```python
from build123d import *

# Parameters (mm, degrees)
BLANKSKE_W         = 44.45
BLANKSKE_H         = 10.795
BLANK_DEPTH        = 9.525
TOOTHCUTSIM_DEPTH  = 47.723229233
TEETHCUTS_COUNT    = 12
TEETHCUTS_PITCH    = 3.989822666
SKETCH1_R          = 2.4892
CUT_EXTRUDE1_DEPTH = 14.478


with BuildPart() as part:
    # BlankSke → Blank (new body)
    with BuildSketch(Plane.XY):
        with Locations((22.225, 5.3975)):
            Rectangle(BLANKSKE_W, BLANKSKE_H)
    extrude(amount=-BLANK_DEPTH)

    # TooCutSkeSim → ToothCutSim (cut, through all)
    with BuildSketch(Plane.XY):
        Polygon((0.595165029, 8.001), (-0.595165029, 8.001), (-1.621342708, 10.8204), (1.621342708, 10.8204), align=None)
    toothcutsim = extrude(amount=-TOOTHCUTSIM_DEPTH, mode=Mode.SUBTRACT)

    # TeethCuts: ToothCutSim ×12
    with Locations(*[(i * TEETHCUTS_PITCH, 0, 0) for i in range(1, TEETHCUTS_COUNT)]):
        add(toothcutsim, mode=Mode.SUBTRACT)

    # Sketch1 → Cut-Extrude1 (cut)
    with BuildSketch(Plane.XY):
        with Locations((5.08, 4.0005)):
            Circle(SKETCH1_R)
    extrude(amount=-CUT_EXTRUDE1_DEPTH, mode=Mode.SUBTRACT)


solid = part.part
```
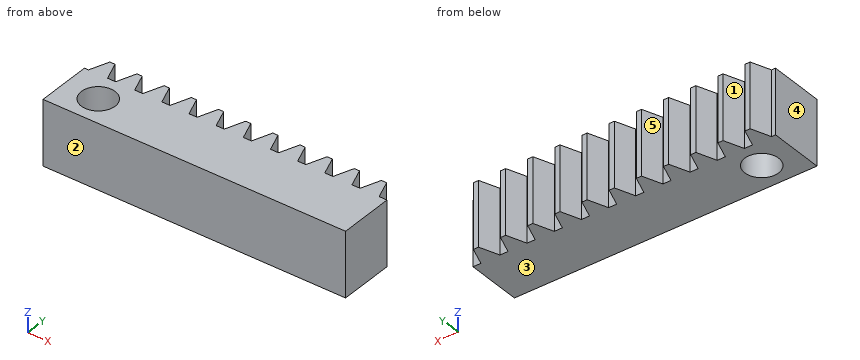
Source: CAD feature listing. Evaluate the final solid. Frame: model axes, mm. Face numbers are marked on the shaded views. A direction names the side the tool comes from. Give positions to 0.01 mm unless a question says otherwise; leave off trailing zeros. Write each loop counter-clockwise with the first axis right and the second up, starting at its lowest first coordinate (ties: lowest second). Pieces come first, ordered by that corner, then holes.
1. Access query for the marked faces 1 and 2. Directions: +Z, -Z, +X, -X, +Y, -Y. A direction counts if a zero-diameter tool reaches every point of the face in a straight line with its end or side. Return the directions, or none.
2. Section query C-C (y = 10). Count the separate pieces of the cut face and the enclosed holes in it, then the cut area to 3 significant figures.
3. Section query B-B (y = 4.5). Return the cut outline in (x, z) (3 decimals), then the cut area to 3 significant figures.
4. Material intervals for line 1 along X through (y, z) = (4, -0.5); line 2 along X through (y, z) = (5.75, -5.25); line 3 along Y through (x, z) = (27.5, -1), sorted ascending.
5. First-contact query: pin 1 (1 mm diameter, centred on x = 37, z = -3, fed in from -Y); pin 2 (0.6 mm diameter, centred on x = 16, z = -4.5, fed in from +Y). Flat tips, straight axial feed; report the tip coordinate or a pass-through.
6. Section query A-A (x = 4). Return the cut outline in (y, z) (3 decimals).
7. Pull-direction query (X, two-part tool) for the marked faces 3, 4 and 5; classes: +X half, -X half, draft (parallel to the pull), parting line (faces both ways), or undercut.
Output values:
1. face 1: +Z, -Z, +Y
1. face 2: +Z, -Z, +X, -X, -Y
2. separate pieces: 11
2. enclosed holes: 0
2. area: 141 mm2
3. outline: (0, -9.525) - (2.641, -9.525) - (2.641, 0) - (0, 0) - close; (7.519, -9.525) - (44.45, -9.525) - (44.45, 0) - (7.519, 0) - close
3. area: 377 mm2
4. line 1: x = 0 to 2.59, 7.57 to 44.45
4. line 2: x = 0 to 3.31, 6.85 to 44.45
4. line 3: y = 0 to 8
5. pin 1: stops at y = 0
5. pin 2: stops at y = 8
6. outline: (0, -9.525) - (1.758, -9.525) - (1.758, 0) - (0, 0) - close; (6.243, -9.525) - (8.001, -9.525) - (8.001, 0) - (6.243, 0) - close
7. face 3: draft
7. face 4: -X half
7. face 5: undercut
